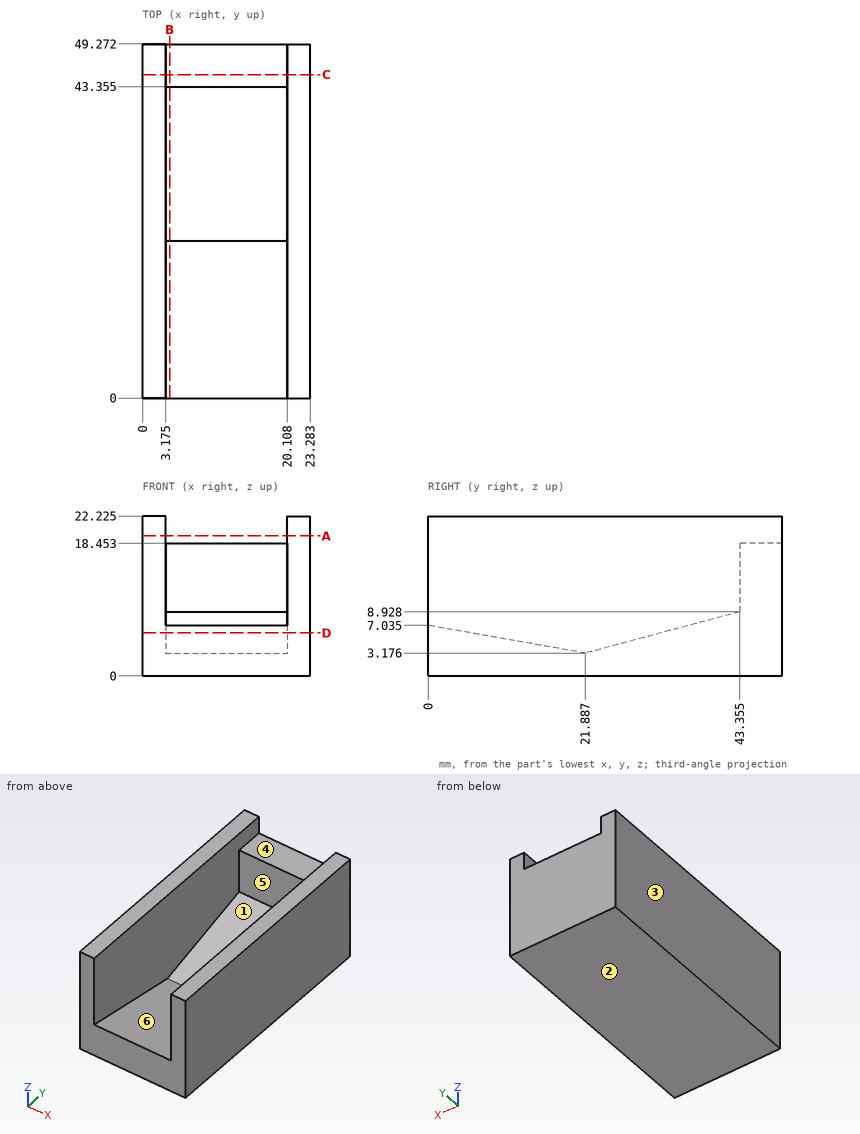
Can you work these out from the drawing? Everything is in mm from the part's minimum corner. A direction names the side the tool comes from. Round coordinates to 2 decimals unless told otherwise and drop trailing zeros. Order: outer loops, then holes, each group sorted by start corner. A loop starts at its lowest first (then second) coordinate and runs counter-clockwise, first axis right, second up. Notation, with made-up numbers: (10, 0) - (51, 0) arc R22 cw to (51, 33) - close; hole circle Ø7 at (65, -15). An arc over 180 degrees is marked (long way). Answer in a Markdown table with one row per item.
(1) Suppose I cut it at D-D, the plane z = 6. Please give me the cut outline in (x, y) (1 decimal).
From the geometry:
| item | result |
|---|---|
| outline | (0, 0) - (23.3, 0) - (23.3, 49.3) - (0, 49.3) - close; hole (3.2, 5.9) - (20.1, 5.9) - (20.1, 32.4) - (3.2, 32.4) - close |
(2) Which directions (+Z, -Z, +X, -X, +Y, -Y) give clear straight access to the entire face, cutting with the end or side of a thin tool? Please do the marked faces 4, 5 and 6.
From the geometry:
| item | result |
|---|---|
| face 4 | +Z, +Y, -Y |
| face 5 | +Z, -Y |
| face 6 | +Z |
(3) For P1, Ø5, axis at x = 10.5, z = 15, coming from the -Y side (3 decimals); P2, Ø1, axis at x = 6.5, y = 34.5, coming from the +Z side; P3, Ø2, axis at x = 10.5, y = 17.5, coming from the +Z side, each with a flat end and sliding along its axis, tell me the tip position at first contact or that it passes through.
From the geometry:
| item | result |
|---|---|
| P1 | stops at y = 43.355 |
| P2 | stops at z = 6.69 |
| P3 | stops at z = 4.13 |
(4) Suppose I cut it at C-C, the plane y = 45. Please give me the cut outline in (x, z) (1 decimal), plus the area to 3 significant figures.
From the geometry:
| item | result |
|---|---|
| outline | (0, 0) - (23.3, 0) - (23.3, 22.2) - (20.1, 22.2) - (20.1, 18.5) - (3.2, 18.5) - (3.2, 22.2) - (0, 22.2) - close |
| area | 454 mm2 |
(5) If we mould it in two halves opening along X, with no side actions, what happens to the marked faces 1, 2 and 3? For each: released by +X, released by -X, zero draft, split by the parting line, or undercut.
From the geometry:
| item | result |
|---|---|
| face 1 | undercut |
| face 2 | zero draft |
| face 3 | released by -X |
(6) Suppose I cut it at A-A, the plane z = 19.5. Please give me the cut outline in (x, y) (1 decimal).
From the geometry:
| item | result |
|---|---|
| outline | (0, 0) - (3.2, 0) - (3.2, 49.3) - (0, 49.3) - close; (20.1, 0) - (23.3, 0) - (23.3, 49.3) - (20.1, 49.3) - close |
(7) Suppose I cut it at B-B, the plane x = 3.75. Please give me the cut outline in (y, z) (1 decimal).
From the geometry:
| item | result |
|---|---|
| outline | (0, 0) - (49.3, 0) - (49.3, 18.5) - (43.4, 18.5) - (43.4, 8.9) - (21.9, 3.2) - (0, 7) - close |
(8) Please list where these lines run through material, in increasing order: L1, parallel to X at y = 26.5, z = 11.25 (1 decimal); L2, parallel to Y at x = 20, z = 14.25 (1 decimal); L3, parallel to Z at x = 14.75, y = 8.5. Write a range as from..to.
From the geometry:
| item | result |
|---|---|
| L1 | x = 0..3.2, 20.1..23.3 |
| L2 | y = 43.4..49.3 |
| L3 | z = 0..5.54 |
